```python
from build123d import *

# Parameters (mm, degrees)
BOSS_EXTRUDE1_DEPTH = 20
CUT_EXTRUDE1_REACH  = 374.693
SKETCH2_R           = 4
CUT_EXTRUDE2_DEPTH  = 20


with BuildPart() as part:
    # Sketch1 → Boss-Extrude1 (new body)
    with BuildSketch(Plane.XY):
        Polygon((0, -10), (34.588658989, -10), (140, -160.542996553), (140, -190), (160, -190), (160, -154.237020775), (45, 10), (0, 10), (-45, 10), (-160, -154.237020775), (-160, -190), (-140, -190), (-140, -160.542996553), (-34.588658989, -10), align=None)
    extrude(amount=BOSS_EXTRUDE1_DEPTH)

    # Cut-Extrude1: up to this face of the body (flat: up to its plane)
    cut_extrude1_end = Plane(part.part.faces().sort_by_distance((-160, -172.118510388, 10))[0])
    # Sketch2 → Cut-Extrude1 (cut, up to the picked face)
    with BuildSketch(Plane(origin=(160, 0, 0), x_dir=(0, 0, -1), z_dir=(1, 0, 0)), mode=Mode.PRIVATE) as cut_extrude1_sk1:
        with Locations(Location((-10, -175, 0), (0, 0, 90))):
            Circle(SKETCH2_R)
    cut_extrude1_tool1 = split(extrude(cut_extrude1_sk1.sketch, amount=-CUT_EXTRUDE1_REACH, mode=Mode.PRIVATE), bisect_by=cut_extrude1_end, keep=Keep.BOTH, mode=Mode.PRIVATE)
    add(cut_extrude1_tool1.solids().sort_by(Axis((160, -175, 10), (-1, 0, 0)))[0], mode=Mode.SUBTRACT)

    # Sketch3 → Cut-Extrude2 (cut)
    with BuildSketch(Plane(origin=(0, 10, 0), x_dir=(1, 0, 0), z_dir=(0, 1, 0))):
        with BuildLine():
            ThreePointArc((3, -10), (2.121320344, -7.878679656), (0, -7))
            Line((0, -7), (0, -10))
            Line((0, -10), (3, -10))
        make_face()
        with BuildLine():
            Line((0, -10), (0, -7))
            ThreePointArc((0, -7), (-2.121320344, -7.878679656), (-3, -10))
            Line((-3, -10), (0, -10))
        make_face()
        with BuildLine():
            Line((3, -10), (0, -10))
            Line((0, -10), (0, -13))
            ThreePointArc((0, -13), (2.121320344, -12.121320344), (3, -10))
        make_face()
        with BuildLine():
            Line((0, -13), (0, -10))
            Line((0, -10), (-3, -10))
            ThreePointArc((-3, -10), (-2.121320344, -12.121320344), (0, -13))
        make_face()
    extrude(amount=-CUT_EXTRUDE2_DEPTH, mode=Mode.SUBTRACT)


solid = part.part
```
Design review of the part built by this model. Coordinates are the model's own, in mm. A direction names the side the tool comes from. Coordinates: 2 decimals unless noted, no trailing zeros. Loops run counter-clockwise (first coordinate to the right, second up) from the corner with the lowest first, then second, coordinate; pieces in that order, holes last. Notation, with made-up numbers: (21.5, 51) - (51.5, 51) arc R28 ccw to (51.5, 89) - close; hole circle Ø7 at (-25.75, 80.25). An arc over 180 degrees is marked (long way). Use CSV: the item, a comma, the result in double quotes. Start each with the question number.
1) Wall thickness on L1, parallel to Z at x = -153, y = -175; L2, parallel to X at y = -131, z = 10.75; L3, parallel to X at y = -58, z = 3.75: over which ranges is each line inside the solid? List them lowest first. Write a range as from..to.
2) Consider section D-D on x = 132. Write out the cut boundary in (y, z).
3) Consider section B-B on y = -146. Write out the cut boundary in (x, z), then the cut area to 3 significant figures.
4) Consider section C-C on y = -2. Write out the cut boundary in (x, z), then the cut area to 3 significant figures.
5) Tool access review of faces 1 (the flat face through (160, -168, 10)), 2 (the flat face through (86.56, -84.22, 9.86)): name each direction out of +Z, -Z, +X, -X, +Y, -Y from which nothing blocks a thin tool from reaching the whole face with its end or side.
6) For pin 1 Ø1 at (y, z) = (-17.5, 2.5) entering from -X; pin 2 Ø10 at (x, z) = (80.5, 9.5) entering from -Y; pin 3 Ø5 at (y, z) = (-124.5, 17) entering from -X, all flat-tipped, find the tip position at first contact; note any pin that passes through.
7) Consider section A-A on y = -175. Write out the cut boundary in (x, z).
8) The part is to be moulded in two halves that separate along Y. For faces 3 (the flat face through (-101.695, -70.969, 9.86)), 4 (the cylindrical face through (150.14, -171.185, 11.201)), 5 (the cylindrical face through (-149.86, -171.185, 11.201)), 6 (the flat face through (-140, -179, 8)), say which applies: +Y half, -Y half, draft (parallel to the pull), parting line (faces both ways), or undercut.
Geometry says:
1,L1,"0..6, 14..20"
1,L2,"-143.73..-119.31, 119.31..143.73"
1,L3,"-92.61..-68.2, 68.2..92.61"
2,outline,"(-149.12, 0) - (-114.25, 0) - (-114.25, 20) - (-149.12, 20) - close"
3,outline,"(-154.23, 0) - (-129.82, 0) - (-129.82, 20) - (-154.23, 20) - close; (129.82, 0) - (154.23, 0) - (154.23, 20) - (129.82, 20) - close"
3,area,"977 mm^2"
4,outline,"(-53.4, 0) - (53.4, 0) - (53.4, 20) - (-53.4, 20) - close; hole circle Ø6 at (0, 10)"
4,area,"2,110 mm^2"
5,face 1,"+Z, -Z, +X, +Y, -Y"
5,face 2,"+Z, -Z, -Y"
6,pin 1,"x = -64.61"
6,pin 2,"y = -82.71"
6,pin 3,"x = -140.93"
7,outline,"(-160, 0) - (-140, 0) - (-140, 6) - (-160, 6) - close; (-160, 14) - (-140, 14) - (-140, 20) - (-160, 20) - close; (140, 0) - (160, 0) - (160, 6) - (140, 6) - close; (140, 14) - (160, 14) - (160, 20) - (140, 20) - close"
8,face 3,"+Y half"
8,face 4,"undercut"
8,face 5,"undercut"
8,face 6,"draft"
